Job drawing, mm, ordinate dimensions from the low corner. One solid piece. A direction names the side the tool comes from. Give positions to 0.01 mm unless a question says otherwise; leave off trailing zeros. Order: outer loops, then holes, each group sorted by start corner. A loop starts at its lowest first (then second) coordinate and runs counter-clockwise, first axis right, second up.
1. Probe line 1 (Y direction, x = 33, z = 30.5); line 2 (X direction, y = 73, z = 43); line 3 (Z direction, x = 37, y = 48). List the from-to ranges inside material, lowest first.
2. Slice it at C-C on z = 13.5. List the corners of the cut face in (x, y).
3. Slice it at B-B on z = 58. List the corners of the cut face in (x, y), and give its area (3 significant figures).
4. Which spindle directions (+Z, -Z, +X, -X, +Y, -Y) get a long thin tool onto all of the face, cutting with end or side? Do the marked faces 1, 2 and 3. Say none if no direction does.
5. Slice it at A-A on x = 28. List the corners of the cut face in (y, z).
6. Slice it at D-D on y = 54. List the corners of the cut face in (x, z).
7. Mould opens along Y. For the marked faces 4, 5, 6 and 7 say: +Y half, -Y half, draft (parallel to the pull), parting line (faces both ways), or undercut.
8. Drop flat-ended pins along their axis: pin 1 Ø22 at (y, z) = (42.5, 10) entering from -X; pin 2 Ø4.5 at (y, z) = (71.5, 46) entering from +X; pin 3 Ø1.5 at (x, y) = (36, 21) entering from +Z. Give the stop position or say it passes through.
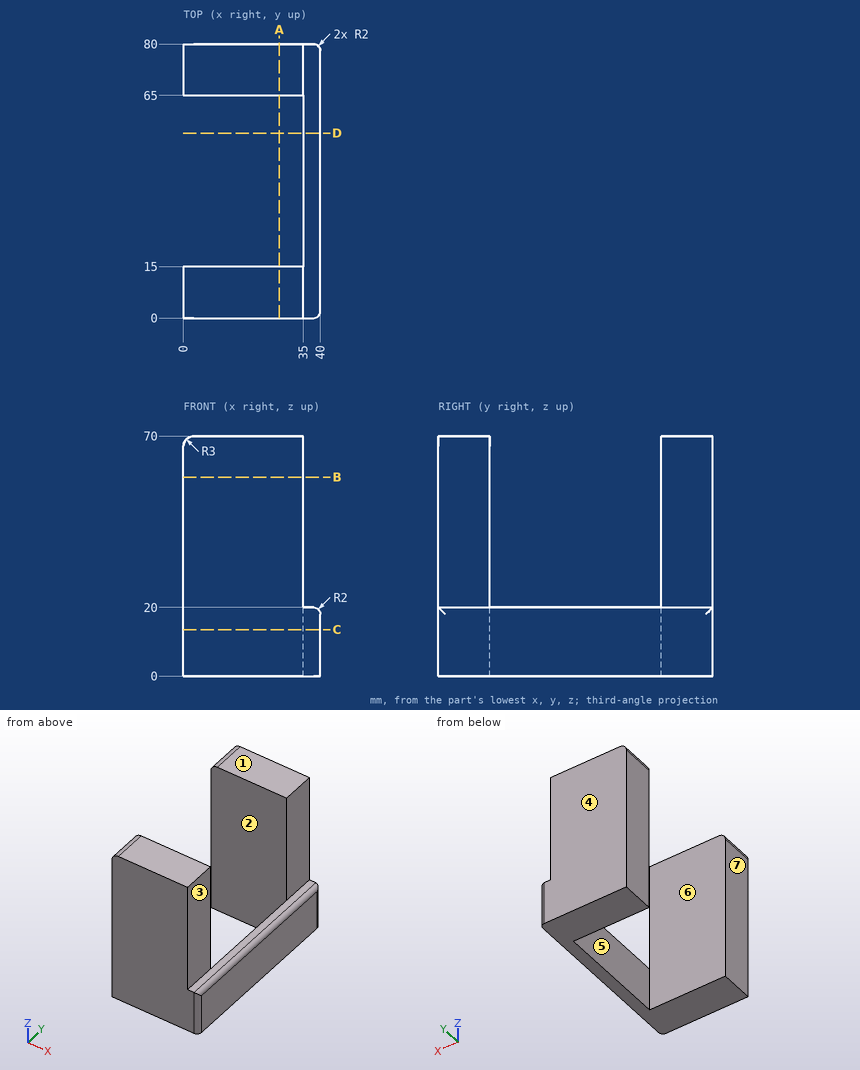
Data:
1. line 1: y = 0 to 15, 65 to 80
1. line 2: x = 0 to 35
1. line 3: z = 0 to 20
2. outline: (0, 0) - (38, 0) arc R2 ccw to (40, 2) - (40, 78) arc R2 ccw to (38, 80) - (0, 80) - (0, 65) - (35, 65) - (35, 15) - (0, 15) - close
3. outline: (0, 0) - (35, 0) - (35, 15) - (0, 15) - close; (0, 65) - (35, 65) - (35, 80) - (0, 80) - close
3. area: 1,050 mm2
4. face 1: +Z, +X, -X, +Y, -Y
4. face 2: +Z, -Z, -X
4. face 3: +Z, +X, +Y, -Y
5. outline: (0, 0) - (15, 0) - (15, 70) - (0, 70) - close; (65, 0) - (80, 0) - (80, 70) - (65, 70) - close
6. outline: (35, 0) - (40, 0) - (40, 18) arc R2 ccw to (38, 20) - (35, 20) - close
7. face 4: +Y half
7. face 5: undercut
7. face 6: undercut
7. face 7: draft
8. pin 1: stops at x = 35
8. pin 2: stops at x = 35
8. pin 3: stops at z = 20
